Build history of the part. All positions in model axes, mm. A direction names the side the tool comes from. Give positions to 0.01 mm unless a question says otherwise; leave off trailing zeros. Order: outer loops, then holes, each group sorted by start corner. A loop starts at its lowest first (then second) coordinate and runs counter-clockwise, first axis right, second up. Notation, with made-up numbers: (32.5, 46) - (39.5, 46) arc R11 ccw to (39.5, 67) - close; hole circle Ø11 at (88.5, 17). An arc over 180 degrees is marked (long way). Use a Markdown table: item, result. Add a question column.
(1) Flat gauge pins, fed straight in: pin 1 (5 mm diameter, centred on x = 7.5, y = -47, fed in from -Z); pin 2 (6 mm diameter, centred on x = -1, y = -26, fed in from -Z); pin 3 (7 mm diameter, centred on x = -0.5, y = -44.5, fed in from -Z). Where does each tip first touch, or does it go through?
(2) Slice it at D-D (z = 12). Write the cut outline in (x, y) (3 decimals), then the cut area to 4 significant figures.
(3) Slice it at B-B (y = -46). Write the cut outline in (x, z) (3 decimals).
(4) Slice it at C-C (x = -7). Write the cut outline in (y, z) (3 decimals).
(5) Which spindle directions (+Z, -Z, +X, -X, +Y, -Y) get a long thin tool onto all of the face, cutting with end or side? Do faces 1 (the face through (0, -46, -8)), 2 (the face through (-0.69, -49.1, -4.96)), 3 (the face through (0, -46, 57)). Say none if no direction does.
(6) Slice it at A-A (z = -4). Write the cut outline in (x, y) (3 decimals), then the cut area to 3 significant figures.
(7) Wall check: line 1 (Y direction, x = 3.75, z = 33.5) (3 decimals); line 2 (Y direction, x = -2, z = -7); line 3 (Z direction, x = -5.75, y = -13.5). Give the ranges that are in metal, low to high.
(8) Mould opens along Y. For faces 4 (the face through (0, -103, 23)), 5 (the face through (0, -96, -2)), 6 (the face through (15, -47, 31)), 7 (the face through (0, -100, -6)) say: +Y half, -Y half, draft (parallel to the pull), parting line (faces both ways), or undercut.
from build123d import *

# Parameters (mm, degrees)
BOSS_EXTRUDE3_DEPTH      = 57
BOSS_EXTRUDE3_DEPTH_BACK = 2
SKETCH1_W                = 30
SKETCH1_H                = 113
SKETCH1_6_R              = 3.175
BOSS_EXTRUDE4_DEPTH      = 8
CUT_EXTRUDE1_DEPTH       = 122.482509029
CUT_EXTRUDE1_DEPTH_BACK  = 122.482509029
SKETCH2_W                = 49
SKETCH2_H                = 42.825
SKETCH2_H_2              = 43.825
SKETCH3_W                = 30
SKETCH3_H                = 3
BOSS_EXTRUDE5_DEPTH      = 8
FILLET2_R                = 10
FILLET3_R                = 10
FILLET4_R                = 5
FILLET5_R                = 5


with BuildPart() as part:
    # Sketch1 → Boss-Extrude3 (new, two sides: drawn at the far end of the back side and taken through both)
    with BuildSketch(Plane.XY.offset(-BOSS_EXTRUDE3_DEPTH_BACK)):
        with Locations((0, -46.5)):
            Rectangle(SKETCH1_W, SKETCH1_H)
    extrude(amount=BOSS_EXTRUDE3_DEPTH + BOSS_EXTRUDE3_DEPTH_BACK)

    # Sketch1<6> → Boss-Extrude4 (add)
    with BuildSketch(Plane.XY):
        with Locations((0, -46)):
            Circle(SKETCH1_6_R)
    extrude(amount=-BOSS_EXTRUDE4_DEPTH)

    # Sketch2 → Cut-Extrude1 (cut, two sides: drawn at the far end of the back side and taken through both)
    with BuildSketch(Plane(origin=(15, 0, 0), x_dir=(0, 0, -1), z_dir=(1, 0, 0)).offset(-CUT_EXTRUDE1_DEPTH_BACK)):
        with Locations((-22.5, -21.4125)):
            Rectangle(SKETCH2_W, SKETCH2_H)
        with Locations((-22.5, -71.0875)):
            Rectangle(SKETCH2_W, SKETCH2_H_2)
    extrude(amount=CUT_EXTRUDE1_DEPTH + CUT_EXTRUDE1_DEPTH_BACK, mode=Mode.SUBTRACT)

    # Sketch3 → Boss-Extrude5 (add)
    with BuildSketch(Plane(origin=(0, 0, -2), x_dir=(-1, 0, 0), z_dir=(0, 0, -1))):
        with Locations((0, 8.5)):
            Rectangle(SKETCH3_W, SKETCH3_H)
        with Locations((0, -101.5)):
            Rectangle(SKETCH3_W, SKETCH3_H)
    extrude(amount=BOSS_EXTRUDE5_DEPTH)

    # Fillet2
    fillet2_edges = [part.edges().sort_by_distance(p)[0] for p in [
        (0, 0, 47),
    ]]
    fillet(fillet2_edges, radius=FILLET2_R)

    # Fillet3
    fillet3_edges = [part.edges().sort_by_distance(p)[0] for p in [
        (0, -93, 47),
    ]]
    fillet(fillet3_edges, radius=FILLET3_R)

    # Fillet4
    fillet4_edges = [part.edges().sort_by_distance(p)[0] for p in [
        (0, -42.825, 47),
    ]]
    fillet(fillet4_edges, radius=FILLET4_R)

    # Fillet5
    fillet5_edges = [part.edges().sort_by_distance(p)[0] for p in [
        (0, -49.175, 47),
    ]]
    fillet(fillet5_edges, radius=FILLET5_R)


solid = part.part
Solution:
| question | item | result |
|---|---|---|
| 1 | pin 1 | z = -2 |
| 1 | pin 2 | z = 47 |
| 1 | pin 3 | z = -8 |
| 2 | outline | (-15, -103) - (15, -103) - (15, -93) - (-15, -93) - close; (-15, -49.175) - (15, -49.175) - (15, -42.825) - (-15, -42.825) - close; (-15, 0) - (15, 0) - (15, 10) - (-15, 10) - close |
| 2 | area | 790.5 mm2 |
| 3 | outline | (-15, -2) - (-3.175, -2) - (-3.175, -8) - (3.175, -8) - (3.175, -2) - (15, -2) - (15, 57) - (-15, 57) - close |
| 4 | outline | (-103, -10) - (-100, -10) - (-100, -2) - (-93, -2) - (-93, 37) arc R10 cw to (-83, 47) - (-54.175, 47) arc R5 cw to (-49.175, 42) - (-49.175, -2) - (-42.825, -2) - (-42.825, 42) arc R5 cw to (-37.825, 47) - (-10, 47) arc R10 cw to (0, 37) - (0, -2) - (7, -2) - (7, -10) - (10, -10) - (10, 57) - (-103, 57) - close |
| 5 | face 1 | -Z, +X, -X |
| 5 | face 2 | -Z |
| 5 | face 3 | +Z, +X, -X, +Y, -Y |
| 6 | outline | (-15, -103) - (15, -103) - (15, -100) - (-15, -100) - close; (-15, 7) - (15, 7) - (15, 10) - (-15, 10) - close; circle Ø6.35 at (0, -46) |
| 6 | area | 212 mm2 |
| 7 | line 1 | -103 to -93, -49.175 to -42.825, 0 to 10 |
| 7 | line 2 | -103 to -100, -48.47 to -43.53, 7 to 10 |
| 7 | line 3 | 47 to 57 |
| 8 | face 4 | -Y half |
| 8 | face 5 | undercut |
| 8 | face 6 | draft |
| 8 | face 7 | undercut |
